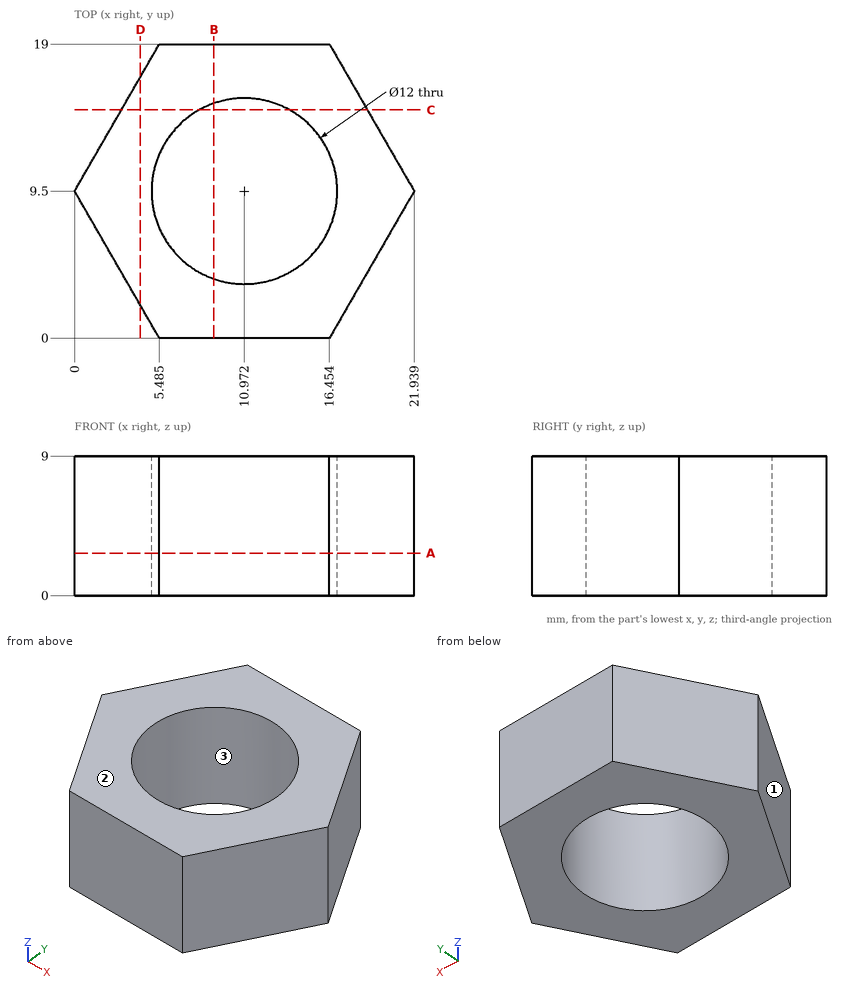
Geometry check sheet. Reference: drawing and pictorial views, mm from the part's lowest x, y, z. Round coordinates to 2 decimals unless told otherwise and drop trailing zeros. Loops run counter-clockwise (first coordinate to the right, second up) from the corner with the lowest first, then second, coordinate; pieces in that order, holes last.
1. Sectioned sample at B-B on x = 9. Record the boundary of the cut face in (y, z).
2. Sectioned sample at D-D on x = 4.25. Record the boundary of the cut face in (y, z), and give its area (4 significant figures).
3. Sectioned sample at A-A on z = 2.75. Record the boundary of the cut face in (x, y) (1 decimal).
4. Sectioned sample at C-C on y = 14.75. Record the boundary of the cut face in (x, z).
5. Mould release check, pull along Y, two halves, no side actions. Record for the marked faces 1, 2 and 3: released by +Y, released by -Y, zero draft, split by the parting line, or undercut.
6. Scan lines: probe 1 along X at (y, z) = (8.25, 4.25) (1 decimal); probe 2 along Y at (x, z) = (5.75, 5.5) (1 decimal); probe 3 along X at (y, z) = (15, 8) (1 decimal). Record each from-to range of solid material in increasing order.
7. Gauge pin test, flat ends, axial feed: pin 1 Ø2 at (x, y) = (7, 4) entering from -Z; pin 2 Ø3 at (y, z) = (17, 1.5) entering from -X (1 decimal); pin 3 Ø1 at (y, z) = (12.5, 8) entering from -X. Record the tip position at first contact, or that the pin passes through.
Recorded:
1. outline: (0, 0) - (3.83, 0) - (3.83, 9) - (0, 9) - close; (15.17, 0) - (19, 0) - (19, 9) - (15.17, 9) - close
2. outline: (2.14, 0) - (16.86, 0) - (16.86, 9) - (2.14, 9) - close
2. area: 132.5 mm2
3. outline: (0, 9.5) - (5.5, 0) - (16.5, 0) - (21.9, 9.5) - (16.5, 19) - (5.5, 19) - close; hole circle Ø12 at (11, 9.5)
4. outline: (3.03, 0) - (8.07, 0) - (8.07, 9) - (3.03, 9) - close; (13.88, 0) - (18.91, 0) - (18.91, 9) - (13.88, 9) - close
5. face 1: released by -Y
5. face 2: zero draft
5. face 3: undercut
6. probe 1: x = 0.7 to 5.1, 16.8 to 21.2
6. probe 2: y = 0 to 6.5, 12.5 to 19
6. probe 3: x = 3.2 to 8.6, 13.4 to 18.8
7. pin 1: stops at z = 0
7. pin 2: stops at x = 3.5
7. pin 3: stops at x = 1.44
